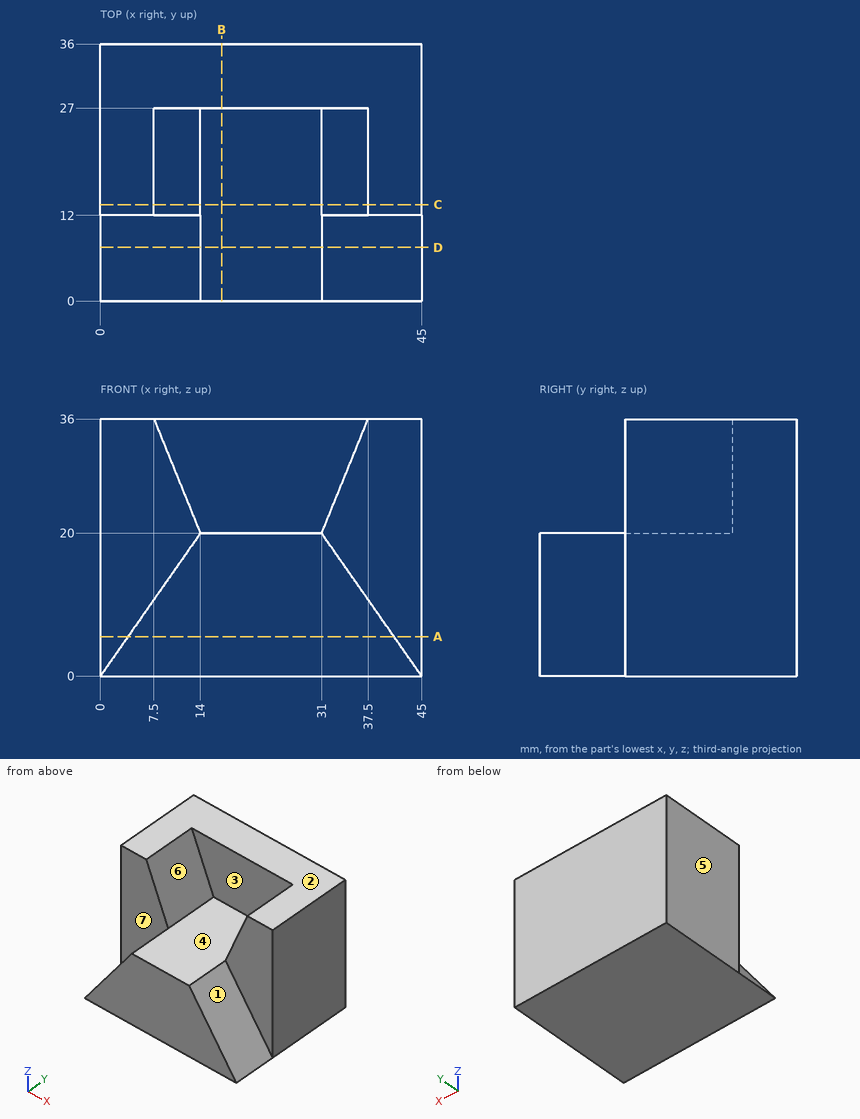
For this review, use the dimensioned drawing (mm, ordinates from the lowest corner) and the shaded views. A direction names the side the tool comes from. Round coordinates to 2 decimals unless told otherwise and drop trailing zeros. Write each loop counter-clockwise with the first axis right and the second up, starting at its lowest first coordinate (ties: lowest second). Pieces come first, ordered by that corner, then holes. Notation, with made-up numbers: (-34.75, 86.25) -> (-4.75, 86.25) arc R27 cw to (-4.75, 115.25) -> close; hole circle Ø3 at (7.25, 44). An arc over 180 degrees is marked (long way). Answer in a Markdown table with one row per item.
Q1. Take a section at D-D, the plane y = 7.5. State the section outline as (x, z) points.
The answers:
| item | result |
|---|---|
| outline | (0, 0) -> (45, 0) -> (31, 20) -> (14, 20) -> close |
Q2. Take a section at B-B, the plane x = 17. State the section outline as (y, z) points.
The answers:
| item | result |
|---|---|
| outline | (0, 0) -> (36, 0) -> (36, 36) -> (27, 36) -> (27, 20) -> (0, 20) -> close |
Q3. Take a section at C-C, the plane y = 13.5. State the section outline as (x, z) points, then the cut area to 3 significant figures.
The answers:
| item | result |
|---|---|
| outline | (0, 0) -> (45, 0) -> (45, 36) -> (37.5, 36) -> (31, 20) -> (14, 20) -> (7.5, 36) -> (0, 36) -> close |
| area | 1,240 mm² |
Q4. For the marked faces 1, 2 and 3, list the 3-axis set-ups (+Z, -Z, +X, -X, +Y, -Y) from which the entire face can be reached by the end or side of a thin tool; tool diameter is ignored.
The answers:
| item | result |
|---|---|
| face 1 | +Z, +X, -Y |
| face 2 | +Z, +X, -X, +Y, -Y |
| face 3 | +Z, -Y |
Q5. Clearance check with flat-ended pins moving along their axes: pin 1 Ø4 at (x, z) = (35.5, 25) entering from -Y; pin 2 Ø8 at (x, z) = (16.5, 26) entering from -Y; pin 3 Ø3 at (x, y) = (16.5, 22) entering from +Z. State where each tip first meets the part, or that it passes through.
The answers:
| item | result |
|---|---|
| pin 1 | y = 12 |
| pin 2 | y = 27 |
| pin 3 | z = 20 |
Q6. Draft analysis for pull direction X (two halves, no side actions). For the marked faces 4, 5, 6 and 7, state which applies: +X half, -X half, draft (parallel to the pull), parting line (faces both ways), or undercut.
The answers:
| item | result |
|---|---|
| face 4 | undercut |
| face 5 | -X half |
| face 6 | undercut |
| face 7 | draft |
Q7. Take a section at A-A, the plane z = 5.5. State the section outline as (x, y) points.
The answers:
| item | result |
|---|---|
| outline | (0, 12) -> (3.85, 12) -> (3.85, 0) -> (41.15, 0) -> (41.15, 12) -> (45, 12) -> (45, 36) -> (0, 36) -> close |
Q8. To check wall thickness, follow L1, parallel to Z at x = 26.5, y = 26; L2, parallel to Y at x = 14, z = 34.5; L3, parallel to X at y = 13.5, z = 23. State the ranges of each line that lie inside material, in increasing order. Write a range as [from, to].
The answers:
| item | result |
|---|---|
| L1 | [0, 20] |
| L2 | [27, 36] |
| L3 | [0, 12.78], [32.22, 45] |
